Read the model definition and answer for the solid it produces. Units are mm, in the model's axes. A direction names the side the tool comes from. Round coordinates to 2 decimals unless told otherwise and drop trailing zeros. Order: outer loops, then holes, each group sorted by start corner. A loop starts at its lowest first (then second) coordinate and runs counter-clockwise, first axis right, second up. Notation, with made-up numbers: (-16.5, 20.25) -> (18.5, 20.25) arc R22 cw to (18.5, 43.25) -> close; hole circle Ø8 at (7, -4). An arc over 180 degrees is marked (long way). Answer as a JSON object with one key per item and string values. Group by question number.
Item 1: For faces 3 (the flat face through (3, -19, 2.67)), 4 (the flat face through (4, -6.5, -5.6)), 5 (the flat face through (20, 0, -0.6)), 6 (the flat face through (7, 0, 14)), determine the directions among +Z, -Z, +X, -X, +Y, -Y from which every point of the face is accessible in a straight line to the end or side of a thin tool.
Item 2: Given P1, Ø14.5, axis at y = -8.5, z = -0.5, coming from the -X side; P2, Ø1.6, axis at x = 2, y = 12, coming from the +Z side; P3, Ø1.2, axis at x = 1, z = -7.5, coming from the +Y side; P4, Ø0.8, axis at y = -6, z = 6, coming from the +X side, each flat-ended and moving along its own axis, determine where each tip first touches the part or whether it passes through.
Item 3: Consider probe 1 along X at (y, z) = (-12, 0.5); probe 2 along X at (y, z) = (10, 15); probe 3 along Y at (x, z) = (15.25, -0.5). Determine where each line is inside the solid, lowest interval first. Write a range as from..to.
Item 4: Section A-A, the plane z = 0 is taken. Write down the section's boundary in (x, y), plus the area to 3 significant figures.
Item 5: Section C-C, the plane x = 15.75 is taken. Write down the section's boundary in (y, z).
Item 6: Section D-D, the plane z = -14 is taken. Write down the section's boundary in (x, y).
Item 7: Section B-B, the plane y = 0 is taken. Write down the section's boundary in (x, z).
Item 8: The mould has two halves that part along Z. Classify faces 1 (the flat face through (1.5, -6.5, -6.512)), 2 (the flat face through (22.5, 0, -2)): pulls with the +Z half, pulls with the -Z half, needs draft (parallel to the pull), parting line crosses it, or undercut.
from build123d import *

# Parameters (mm, degrees)
SKETCH1_R           = 22
BOSS_EXTRUDE1_DEPTH = 10
CUT_EXTRUDE2_DEPTH  = 5.5
SKETCH15_W          = 18
SKETCH15_H          = 24.118038922
CUT_EXTRUDE3_DEPTH  = 3
SKETCH16_R          = 4
BOSS_EXTRUDE2_DEPTH = 12.5
CUT_EXTRUDE4_START  = 22.5
SKETCH8_W           = 1.2
SKETCH8_H           = 10
CUT_EXTRUDE4_DEPTH  = 5
SKETCH17_W          = 4
SKETCH17_H          = 1.75
BOSS_EXTRUDE3_DEPTH = 1
SKETCH18_W          = 4.25
SKETCH18_H          = 1.737607108
BOSS_EXTRUDE4_DEPTH = 1
SKETCH22_R          = 1.5
CUT_EXTRUDE7_DEPTH  = 7


with BuildPart() as part:
    # Sketch1 → Boss-Extrude1 (new body)
    with BuildSketch(Plane(origin=(0, 0, 0), x_dir=(0, 0, -1), z_dir=(1, 0, 0))):
        Circle(SKETCH1_R)
    extrude(amount=BOSS_EXTRUDE1_DEPTH)

    # Sketch13 → Cut-Extrude2 (cut)
    with BuildSketch(Plane(origin=(0, 0, 0), x_dir=(0, 0, -1), z_dir=(1, 0, 0))):
        with BuildLine():
            Line((-2.670420152, -16.85816067), (-2.670420152, -16.530371213))
            Line((-2.670420152, -16.530371213), (-4.762392892, -10))
            Line((-4.762392892, -10), (-4.762392892, -6.943148259))
            Line((-4.762392892, -6.943148259), (-6.5, -6.943148259))
            Line((-6.5, -6.943148259), (-6.5, 19.556851741))
            Line((-6.5, 19.556851741), (6.5, 19.556851741))
            Line((6.5, 19.556851741), (6.5, -6.943148259))
            Line((6.5, -6.943148259), (4.762392892, -6.943148259))
            Line((4.762392892, -6.943148259), (4.762392892, -10))
            Line((4.762392892, -10), (2.670420152, -16.530371213))
            Line((2.670420152, -16.530371213), (2.670420152, -16.85816067))
            Line((2.670420152, -16.85816067), (2.670420152, -21.837327131))
            ThreePointArc((2.670420152, -21.837327131), (1.836835043, -21.92318492), (1.000584871, -21.977234355))
            Line((1.000584871, -21.977234355), (0, -25.25))
            Line((0, -25.25), (-1.000584871, -21.977234355))
            ThreePointArc((-1.000584871, -21.977234355), (-1.836835043, -21.92318492), (-2.670420152, -21.837327131))
            Line((-2.670420152, -21.837327131), (-2.670420152, -16.85816067))
        make_face()
    extrude(amount=CUT_EXTRUDE2_DEPTH, mode=Mode.SUBTRACT)

    # Sketch15 → Cut-Extrude3 (cut)
    with BuildSketch(Plane.ZY):
        with Locations((0, 5.115871202)):
            Rectangle(SKETCH15_W, SKETCH15_H)
    extrude(amount=-CUT_EXTRUDE3_DEPTH, mode=Mode.SUBTRACT)

    # Sketch16 → Boss-Extrude2 (add)
    with BuildSketch(Plane(origin=(10, 0, 0), x_dir=(0, 0, -1), z_dir=(1, 0, 0))):
        Circle(SKETCH16_R)
    extrude(amount=BOSS_EXTRUDE2_DEPTH)

    # Sketch8 → Cut-Extrude4 (cut)
    with BuildSketch(Plane(origin=(0, 0, 0), x_dir=(0, 0, -1), z_dir=(1, 0, 0)).offset(CUT_EXTRUDE4_START)):
        Rectangle(SKETCH8_W, SKETCH8_H)
    extrude(amount=-CUT_EXTRUDE4_DEPTH, mode=Mode.SUBTRACT)

    # Sketch17 → Boss-Extrude3 (add)
    with BuildSketch(Plane(origin=(0, -6.943148259, 0), x_dir=(1, 0, 0), z_dir=(0, 1, 0))):
        with Locations((2, 5.637392892)):
            Rectangle(SKETCH17_W, SKETCH17_H)
    extrude(amount=BOSS_EXTRUDE3_DEPTH)

    # Sketch18 → Boss-Extrude4 (add)
    with BuildSketch(Plane(origin=(0, -6.943148259, 0), x_dir=(1, 0, 0), z_dir=(0, 1, 0))):
        with Locations((2.125, -5.631196446)):
            Rectangle(SKETCH18_W, SKETCH18_H)
    extrude(amount=BOSS_EXTRUDE4_DEPTH)

    # Sketch22 → Cut-Extrude7 (cut)
    with BuildSketch(Plane(origin=(0, 0, 0), x_dir=(0, 0, -1), z_dir=(1, 0, 0))):
        with Locations((-14, 0)):
            Circle(SKETCH22_R)
        with Locations((14, 0)):
            Circle(SKETCH22_R)
    extrude(amount=CUT_EXTRUDE7_DEPTH, mode=Mode.SUBTRACT)


solid = part.part
Values found:
{
 "1": {"face 3": "-X, -Y", "face 4": "none", "face 5": "+X, +Y, -Y", "face 6": "-X"},
 "2": {"P1": "x = 0", "P2": "z = 18.94", "P3": "y = 20.89", "P4": "x = 10"},
 "3": {"probe 1": "5.5..10", "probe 2": "0..10", "probe 3": "-3.97..3.97"},
 "4": {"outline": "(0, 19.56) -> (5.5, 19.56) -> (5.5, -22) -> (10, -22) -> (10, -4) -> (17.5, -4) -> (17.5, 4) -> (10, 4) -> (10, 22) -> (0, 22) -> close", "area": "271 mm2"},
 "5": {"outline": "circle Ø8 at (0, 0)"},
 "6": {"outline": "(0, -16.97) -> (10, -16.97) -> (10, 16.97) -> (0, 16.97) -> (0, 1.5) -> (7, 1.5) -> (7, -1.5) -> (0, -1.5) -> close"},
 "7": {"outline": "(0, -22) -> (10, -22) -> (10, -4) -> (22.5, -4) -> (22.5, -0.6) -> (17.5, -0.6) -> (17.5, 0.6) -> (22.5, 0.6) -> (22.5, 4) -> (10, 4) -> (10, 22) -> (0, 22) -> (0, 15.5) -> (7, 15.5) -> (7, 12.5) -> (0, 12.5) -> (0, 9) -> (3, 9) -> (3, 6.5) -> (5.5, 6.5) -> (5.5, -6.5) -> (3, -6.5) -> (3, -9) -> (0, -9) -> (0, -12.5) -> (7, -12.5) -> (7, -15.5) -> (0, -15.5) -> close"},
 "8": {"face 1": "undercut", "face 2": "needs draft"}
}
